```python
from build123d import *

# Parameters (mm, degrees)
F0_W     = 101.6
F0_H     = 76.2
F1_DEPTH = 4.7625
F2_W     = 38.1
F2_H     = 38.1
F3_DEPTH = 25.4
F4_R     = 3.175
F5_DEPTH = 25.4


with BuildPart() as f1:
    # F0 (on Top) → F1 (new body)
    with BuildSketch(Plane.XY):
        with Locations((50.8, 38.1)):
            Rectangle(F0_W, F0_H)
    extrude(amount=F1_DEPTH)

    # F2 (on face) → F3 (cut)
    with BuildSketch(Plane.XY.offset(4.7625)):
        with Locations((82.55, 19.05)):
            Rectangle(F2_W, F2_H)
        with Locations((19.05, 19.05)):
            Rectangle(F2_W, F2_H)
    extrude(amount=-F3_DEPTH, mode=Mode.SUBTRACT)

    # F4 (on face) → F5 (cut)
    with BuildSketch(Plane.XY.offset(4.7625)):
        with Locations((50.8, 12.7)):
            Circle(F4_R)
        with Locations((50.8, 31.75)):
            Circle(F4_R)
        with Locations((12.7, 57.15)):
            Circle(F4_R)
        with Locations((50.8, 57.15)):
            Circle(F4_R)
        with Locations((88.9, 57.15)):
            Circle(F4_R)
    extrude(amount=-F5_DEPTH, mode=Mode.SUBTRACT)


solid = f1.part
```
Design review of the part built by this model. Coordinates are the model's own, in mm. A direction names the side the tool comes from. Coordinates: 2 decimals unless noted, no trailing zeros. Order: outer loops, then holes, each group sorted by start corner. A loop starts at its lowest first (then second) coordinate and runs counter-clockwise, first axis right, second up.
1) Take a section at A-A, the plane x = 50.8. Give the boundary of the cut face in (y, z) (1 decimal), and give its area (3 significant figures).
2) Mouldability with a two-part tool opening along X and no side actions: class faces 4 (the flat face through (51, 0, 2)), 5 (the cylindrical face through (12.01, 54.05, 2.41)), 6 (the flat face through (0, 57, 2)) as +X half, -X half, draft (parallel to the pull), parting line (faces both ways), or undercut.
3) Take a section at B-B, the plane y = 57.15. Give the boundary of the cut face in (x, z) (1 decimal).
4) Wall thickness on line 1 along Y through (x, z) = (50.8, 1.2) (3 decimals); line 2 along Y through (x, z) = (51.5, 0.55); line 3 along Y through (x, z) = (88.9, 3.6) (3 decimals): over which ranges is each line inside the solid? List them lowest first.
5) Take a section at D-D, the plane y = 12.7. Give the boundary of the cut face in (x, z) (1 decimal), and give its area (3 significant figures).
6) Clearance check with flat-ended pins moving along their axes: pin 1 (1.5 mm diameter, centred on x = 32, z = 3, fed in from -Y); pin 2 (1.5 mm diameter, centred on x = 54.5, y = 44.5, fed in from -Z). State where each tip first meets the part, or that it passes through.
7) For faces 1 (the flat face through (19, 38.1, 2)), 2 (the cylindrical face through (88.21, 54.05, 2.41)), 3 (the flat face through (82, 38.1, 2)), list the 3-axis set-ups (+Z, -Z, +X, -X, +Y, -Y) from which the entire face can be reached by the end or side of a thin tool; tool diameter is ignored.
8) Take a section at C-C, the plane z = 3.7. Give the boundary of the cut face in (x, y) (3 decimals), and give its area (3 significant figures).
Returned:
1. outline: (0, 0) - (9.5, 0) - (9.5, 4.8) - (0, 4.8) - close; (15.9, 0) - (28.6, 0) - (28.6, 4.8) - (15.9, 4.8) - close; (34.9, 0) - (54, 0) - (54, 4.8) - (34.9, 4.8) - close; (60.3, 0) - (76.2, 0) - (76.2, 4.8) - (60.3, 4.8) - close
1. area: 272 mm2
2. face 4: draft
2. face 5: undercut
2. face 6: -X half
3. outline: (0, 0) - (9.5, 0) - (9.5, 4.8) - (0, 4.8) - close; (15.9, 0) - (47.6, 0) - (47.6, 4.8) - (15.9, 4.8) - close; (54, 0) - (85.7, 0) - (85.7, 4.8) - (54, 4.8) - close; (92.1, 0) - (101.6, 0) - (101.6, 4.8) - (92.1, 4.8) - close
4. line 1: y = 0 to 9.525, 15.875 to 28.575, 34.925 to 53.975, 60.325 to 76.2
4. line 2: y = 0 to 9.6, 15.8 to 28.65, 34.85 to 54.05, 60.25 to 76.2
4. line 3: y = 38.1 to 53.975, 60.325 to 76.2
5. outline: (38.1, 0) - (47.6, 0) - (47.6, 4.8) - (38.1, 4.8) - close; (54, 0) - (63.5, 0) - (63.5, 4.8) - (54, 4.8) - close
5. area: 90.7 mm2
6. pin 1: stops at y = 38.1
6. pin 2: stops at z = 0
7. face 1: +Z, -Z, -X, -Y
7. face 2: +Z, -Z
7. face 3: +Z, -Z, +X, -Y
8. outline: (0, 38.1) - (38.1, 38.1) - (38.1, 0) - (63.5, 0) - (63.5, 38.1) - (101.6, 38.1) - (101.6, 76.2) - (0, 76.2) - close; hole circle Ø6.35 at (12.7, 57.15); hole circle Ø6.35 at (50.8, 12.7); hole circle Ø6.35 at (50.8, 31.75); hole circle Ø6.35 at (50.8, 57.15); hole circle Ø6.35 at (88.9, 57.15)
8. area: 4,680 mm2
